Verification items for the finished model (mm, model axes). A direction names the side the tool comes from. Give positions to 0.01 mm unless a question says otherwise; leave off trailing zeros. Order: outer loops, then holes, each group sorted by start corner. A loop starts at its lowest first (then second) coordinate and runs counter-clockwise, first axis right, second up. Notation, with made-up numbers: (39.25, -11.5) -> (62.25, -11.5) arc R36 ccw to (62.25, 23.5) -> close; hole circle Ø10 at (-38, 42.25). An arc over 180 degrees is marked (long way). Write each question's results on one line, items separated by ' | '. Start each with the question number.
1. Material ranges on L1, parallel to X at y = 84, z = 10; L2, parallel to Z at x = 135, y = 82.7; L3, parallel to X at y = 83.7, z = 14, recorded low to high. Write a range as from..to.
2. Cross-section at C-C, the plane x = 135. Enter the section's corners in (y, z).
3. Cross-section at B-B, the plane y = 113.5. Enter the section's corners in (x, z), then the cut area to 3 significant figures.
4. Mould release check, pull along Z, two halves, no side actions. Record for faces 6 (the face through (116.233, 83.268, 4.659)), 7 (the face through (101.039, 127.719, -20.594)), 8 (the face through (139, 106, -3)): +Z half, -Z half, draft (parallel to the pull), parting line (faces both ways), or undercut.
5. Cross-section at D-D, the plane z = 6. Enter the section's corners in (x, y).
6. Depth check by flat-ended pin: pin 1 Ø8 at (x, z) = (135, 6) entering from +Y; pin 2 Ø1.5 at (x, y) = (92.5, 122.5) entering from +Z; pin 3 Ø1.5 at (x, y) = (100.5, 83.5) entering from -Z. Enter the tip coordinate at first touch or a pass-through.
7. Set-up check for faces 1 (the face through (100, 122, -5)), 2 (the face through (125, 123, -21)), 3 (the face through (71.5, 83, 14)), 4 (the face through (63.014, 86.423, -14.499)), 5 (the face through (129, 83, -5)): record each of +Z, -Z, +X, -X, +Y, -Y from which the full face is reachable in a straight line by a thin tool's end or side.
8. Cross-section at A-A, the plane z = -9. Enter the section's corners in (x, y), then the cut area to 3 significant figures.
from build123d import *

# Parameters (mm, degrees)
CYLINDER027_R               = 4
CYLINDER027_DEPTH           = 2.5
CYLINDER027_ROLL_ANGLE      = 90
BOX036_W                    = 14
BOX036_H                    = 10
BOX036_DEPTH                = 11
CYLINDER023_R               = 1.25
CYLINDER023_DEPTH           = 15
CYLINDER023_ROLL_ANGLE      = 90
CYLINDER024_R               = 1.25
CYLINDER024_DEPTH           = 15
CYLINDER024_ROLL_ANGLE      = 90
CYLINDER018_R               = 3.5
CYLINDER018_DEPTH           = 10
CYLINDER019_R               = 3.5
CYLINDER019_DEPTH           = 10
FUSION020_ROLL_ANGLE        = 90
CYLINDER021_R               = 3.5
CYLINDER021_DEPTH           = 10
CYLINDER020_R               = 3.5
CYLINDER020_DEPTH           = 10
FUSION022_ROLL_ANGLE        = 90
BOX018_W                    = 5
BOX018_H                    = 3
BOX018_DEPTH                = 10
BOX035_W                    = 5
BOX035_H                    = 3
BOX035_DEPTH                = 10
BOX025_W                    = 20
BOX025_H                    = 10
BOX025_DEPTH                = 5
BOX024_W                    = 10
BOX024_H                    = 10
BOX024_DEPTH                = 28
FILLET010_R                 = 4.99
BOX022_W                    = 6
BOX022_H                    = 3
BOX022_DEPTH                = 3
CHAMFER002_SIZE             = 2.99
BOX020_W                    = 6
BOX020_H                    = 3
BOX020_DEPTH                = 3
CHAMFER_SIZE                = 2.99
BOX010_W                    = 73
BOX010_H                    = 10
BOX010_DEPTH                = 8
BOX002_W                    = 73
BOX002_H                    = 37
BOX002_DEPTH                = 40
BOX_W                       = 77
BOX_H                       = 48
BOX_DEPTH                   = 40
FILLET_R                    = 8
CYLINDER001_R               = 7
CYLINDER001_DEPTH           = 2
CYLINDER001_PLACEMENT_ANGLE = 29.99999
CYLINDER_R                  = 6
CYLINDER_DEPTH              = 10
CYLINDER_PLACEMENT_ANGLE    = 29.99999
FUSION004_ROLL_ANGLE        = 180
FUSION004_PITCH_ANGLE       = -70
FUSION004_PLACEMENT_ANGLE   = -90


with BuildPart() as cylinder027:
    # Cylinder027 → Cylinder027 (new body)
    with BuildSketch(Plane.XY):
        Circle(CYLINDER027_R)
    extrude(amount=CYLINDER027_DEPTH)


with BuildPart() as cylinder027_1:
    # Cylinder027 roll: moved
    add(cylinder027.part.rotate(Axis((0, 0, 0), (1, 0, 0)), CYLINDER027_ROLL_ANGLE))


with BuildPart() as cylinder027_2:
    # Cylinder027 placement: moved
    add(cylinder027_1.part.moved(Location((63, 84.5, -17))))


with BuildPart() as cube:
    # Box036 → Box036 (new body)
    with BuildSketch(Plane(origin=(129, 78, -10), x_dir=(1, 0, 0), z_dir=(0, 0, 1))):
        with Locations((7, 5)):
            Rectangle(BOX036_W, BOX036_H)
    extrude(amount=BOX036_DEPTH)


with BuildPart() as cylinder023:
    # Cylinder023 → Cylinder023 (new body)
    with BuildSketch(Plane.XY):
        Circle(CYLINDER023_R)
    extrude(amount=CYLINDER023_DEPTH)


with BuildPart() as cylinder023_1:
    # Cylinder023 roll: moved
    add(cylinder023.part.rotate(Axis((0, 0, 0), (1, 0, 0)), CYLINDER023_ROLL_ANGLE))


with BuildPart() as cylinder023_2:
    # Cylinder023 placement: moved
    add(cylinder023_1.part.moved(Location((74, 97, 10))))


with BuildPart() as fusion031:
    # Cylinder024 → Cylinder024 (new body)
    with BuildSketch(Plane.XY):
        Circle(CYLINDER024_R)
    extrude(amount=CYLINDER024_DEPTH)


with BuildPart() as fusion031_1:
    # Cylinder024 roll: moved
    add(fusion031.part.rotate(Axis((0, 0, 0), (1, 0, 0)), CYLINDER024_ROLL_ANGLE))


with BuildPart() as fusion031_2:
    # Cylinder024 placement: moved
    add(fusion031_1.part.moved(Location((106, 97, 10))))

    # Fusion031: union Cylinder023
    add(cylinder023_2.part)


with BuildPart() as fusion031_3:
    # Fusion031 placement: moved
    add(fusion031_2.part.moved(Location((0, -8, 0))))


with BuildPart() as cylinder018:
    # Cylinder018 → Cylinder018 (new body)
    with BuildSketch(Plane(origin=(-8, 25.5, 0), x_dir=(1, 0, 0), z_dir=(0, 0, 1))):
        Circle(CYLINDER018_R)
    extrude(amount=CYLINDER018_DEPTH)


with BuildPart() as fusion020:
    # Cylinder019 → Cylinder019 (new body)
    with BuildSketch(Plane(origin=(-8, 33.5, 0), x_dir=(1, 0, 0), z_dir=(0, 0, 1))):
        Circle(CYLINDER019_R)
    extrude(amount=CYLINDER019_DEPTH)

    # Fusion020: union Cylinder018
    add(cylinder018.part)


with BuildPart() as fusion020_1:
    # Fusion020 roll: moved
    add(fusion020.part.rotate(Axis((0, 0, 0), (1, 0, 0)), FUSION020_ROLL_ANGLE))


with BuildPart() as fusion020_2:
    # Fusion020 placement: moved
    add(fusion020_1.part.moved(Location((312, 84.5, -19.5))))


with BuildPart() as cylinder021:
    # Cylinder021 → Cylinder021 (new body)
    with BuildSketch(Plane(origin=(-8, 25.5, 0), x_dir=(1, 0, 0), z_dir=(0, 0, 1))):
        Circle(CYLINDER021_R)
    extrude(amount=CYLINDER021_DEPTH)


with BuildPart() as fusion023:
    # Cylinder020 → Cylinder020 (new body)
    with BuildSketch(Plane(origin=(-8, 33.5, 0), x_dir=(1, 0, 0), z_dir=(0, 0, 1))):
        Circle(CYLINDER020_R)
    extrude(amount=CYLINDER020_DEPTH)

    # Fusion022: union Cylinder021
    add(cylinder021.part)


with BuildPart() as fusion023_1:
    # Fusion022 roll: moved
    add(fusion023.part.rotate(Axis((0, 0, 0), (1, 0, 0)), FUSION022_ROLL_ANGLE))


with BuildPart() as fusion023_2:
    # Fusion022 placement: moved
    add(fusion023_1.part.moved(Location((334, 84.5, -19.5))))

    # Fusion023: union Fusion020
    add(fusion020_2.part)


with BuildPart() as fusion023_3:
    # Fusion023 placement: moved
    add(fusion023_2.part.moved(Location((-191, 0, 0))))


with BuildPart() as box018:
    # Box018 → Box018 (new body)
    with BuildSketch(Plane(origin=(71.5, 82, 5), x_dir=(1, 0, 0), z_dir=(0, 0, 1))):
        with Locations((2.5, 1.5)):
            Rectangle(BOX018_W, BOX018_H)
    extrude(amount=BOX018_DEPTH)


with BuildPart() as box035:
    # Box035 → Box035 (new body)
    with BuildSketch(Plane(origin=(103.5, 82, 5), x_dir=(1, 0, 0), z_dir=(0, 0, 1))):
        with Locations((2.5, 1.5)):
            Rectangle(BOX035_W, BOX035_H)
    extrude(amount=BOX035_DEPTH)


with BuildPart() as box025:
    # Box025 → Box025 (new body)
    with BuildSketch(Plane(origin=(90, 112, 9), x_dir=(1, 0, 0), z_dir=(0, 0, 1))):
        with Locations((10, 5)):
            Rectangle(BOX025_W, BOX025_H)
    extrude(amount=BOX025_DEPTH)


with BuildPart() as fillet010:
    # Box024 → Box024 (new body)
    with BuildSketch(Plane(origin=(54, 85, -16), x_dir=(1, 0, 0), z_dir=(0, 0, 1))):
        with Locations((5, 5)):
            Rectangle(BOX024_W, BOX024_H)
    extrude(amount=BOX024_DEPTH)

    # Fillet010
    fillet010_edges = [fillet010.edges().sort_by_distance(p)[0] for p in [
        (59, 85, -16),
        (59, 85, 12),
        (59, 95, -16),
        (59, 95, 12),
    ]]
    fillet(fillet010_edges, radius=FILLET010_R)


with BuildPart() as chamfer002:
    # Box022 → Box022 (new body)
    with BuildSketch(Plane(origin=(70, 113, -23), x_dir=(1, 0, 0), z_dir=(0, 0, 1))):
        with Locations((3, 1.5)):
            Rectangle(BOX022_W, BOX022_H)
    extrude(amount=BOX022_DEPTH)

    # Chamfer002
    chamfer002_edges = [chamfer002.edges().sort_by_distance(p)[0] for p in [
        (73, 116, -23),
    ]]
    chamfer(chamfer002_edges, length=CHAMFER002_SIZE)


with BuildPart() as chamfer002_1:
    # Chamfer002 placement: moved
    add(chamfer002.part.moved(Location((55, 9, 0.5))))


with BuildPart() as fusion028:
    # Box020 → Box020 (new body)
    with BuildSketch(Plane(origin=(70, 113, -23), x_dir=(1, 0, 0), z_dir=(0, 0, 1))):
        with Locations((3, 1.5)):
            Rectangle(BOX020_W, BOX020_H)
    extrude(amount=BOX020_DEPTH)

    # Chamfer
    chamfer_edges = [fusion028.edges().sort_by_distance(p)[0] for p in [
        (73, 116, -23),
    ]]
    chamfer(chamfer_edges, length=CHAMFER_SIZE)


with BuildPart() as fusion028_1:
    # Chamfer placement: moved
    add(fusion028.part.moved(Location((1, 9, 0.5))))

    # Fusion028: union Chamfer002
    add(chamfer002_1.part)


with BuildPart() as box010:
    # Box010 → Box010 (new body)
    with BuildSketch(Plane(origin=(64, 82, -23), x_dir=(1, 0, 0), z_dir=(0, 0, 1))):
        with Locations((36.5, 5)):
            Rectangle(BOX010_W, BOX010_H)
    extrude(amount=BOX010_DEPTH)


with BuildPart() as box002:
    # Box002 → Box002 (new body)
    with BuildSketch(Plane(origin=(64, 85, -26), x_dir=(1, 0, 0), z_dir=(0, 0, 1))):
        with Locations((36.5, 18.5)):
            Rectangle(BOX002_W, BOX002_H)
    extrude(amount=BOX002_DEPTH)


with BuildPart() as cut019:
    # Box → Box (new body)
    with BuildSketch(Plane(origin=(62, 82, -27), x_dir=(1, 0, 0), z_dir=(0, 0, 1))):
        with Locations((38.5, 24)):
            Rectangle(BOX_W, BOX_H)
    extrude(amount=BOX_DEPTH)

    # Fillet
    fillet_edges = [cut019.edges().sort_by_distance(p)[0] for p in [
        (100.5, 82, -27),
        (100.5, 82, 13),
        (100.5, 130, -27),
        (100.5, 130, 13),
    ]]
    fillet(fillet_edges, radius=FILLET_R)


with BuildPart() as cut019_1:
    # Fillet placement: moved
    add(cut019.part.moved(Location((0, 0, 4))))

    # Cut001: cut Box002
    add(box002.part, mode=Mode.SUBTRACT)

    # Cut004: cut Box010
    add(box010.part, mode=Mode.SUBTRACT)

    # Cut018: cut Fusion028
    add(fusion028_1.part, mode=Mode.SUBTRACT)

    # Cut019: cut Fillet010
    add(fillet010.part, mode=Mode.SUBTRACT)


with BuildPart() as cylinder001:
    # Cylinder001 → Cylinder001 (new body)
    with BuildSketch(Plane.XY):
        Circle(CYLINDER001_R)
    extrude(amount=CYLINDER001_DEPTH)


with BuildPart() as cylinder001_1:
    # Cylinder001 placement: moved
    add(cylinder001.part.moved(Location((51, 75, -3))).rotate(Axis((51, 75, -3), (0, -1, 0)), CYLINDER001_PLACEMENT_ANGLE))


with BuildPart() as cut025:
    # Cylinder → Cylinder (new body)
    with BuildSketch(Plane.XY):
        Circle(CYLINDER_R)
    extrude(amount=CYLINDER_DEPTH)


with BuildPart() as cut025_1:
    # Cylinder placement: moved
    add(cut025.part.moved(Location((51, 75, -3))).rotate(Axis((51, 75, -3), (0, -1, 0)), CYLINDER_PLACEMENT_ANGLE))

    # Fusion004: union Cylinder001
    add(cylinder001_1.part)


with BuildPart() as cut025_2:
    # Fusion004 roll: moved
    add(cut025_1.part.rotate(Axis((0, 0, 0), (1, 0, 0)), FUSION004_ROLL_ANGLE))


with BuildPart() as cut025_3:
    # Fusion004 pitch: moved
    add(cut025_2.part.rotate(Axis((0, 0, 0), (0, 1, 0)), FUSION004_PITCH_ANGLE))


with BuildPart() as cut025_4:
    # Fusion004 placement: moved
    add(cut025_3.part.moved(Location((175.5, 143.464742, -29.748779))).rotate(Axis((175.5, 143.464742, -29.748779), (0, 0, 1)), FUSION004_PLACEMENT_ANGLE))

    # Fusion029: union Cut019
    add(cut019_1.part)

    # Cut020: cut Box025
    add(box025.part, mode=Mode.SUBTRACT)

    # Fusion030: union Box018, Box035
    add(box018.part)
    add(box035.part)

    # Cut021: cut Fusion023
    add(fusion023_3.part, mode=Mode.SUBTRACT)

    # Cut022: cut Fusion031
    add(fusion031_3.part, mode=Mode.SUBTRACT)

    # Cut023: cut Cube
    add(cube.part, mode=Mode.SUBTRACT)

    # Cut025: cut Cylinder027
    add(cylinder027_2.part, mode=Mode.SUBTRACT)


solid = cut025_4.part
Results below:
1) L1: x = 62..72.75, 75.25..104.75, 107.25..139 | L2: z = -15..-10, 1..2.5, 9.5..10.5 | L3: x = 71.5..76.5, 103.5..108.5
2) outline: (82, -15) -> (85, -15) -> (85, -10) -> (82, -10) -> close; (82, 1) -> (85, 1) -> (85, 14) -> (122, 14) -> (122, -23) arc R8 ccw to (130, -15) -> (130, 9) arc R8 ccw to (122, 17) -> (90, 17) arc R8 ccw to (84.5, 14.81) -> (84.5, 10.5) -> (82.14, 10.5) arc R8 ccw to (82.02, 9.5) -> (84.5, 9.5) -> (84.5, 2.5) -> (82, 2.5) -> close
3) outline: (62, -23) -> (64, -23) -> (64, 14) -> (137, 14) -> (137, -23) -> (139, -23) -> (139, 17) -> (62, 17) -> close | area: 379 mm²
4) face 6: undercut | face 7: -Z half | face 8: draft
5) outline: (62, 82) -> (109.5, 82) -> (109.5, 84.5) -> (116.5, 84.5) -> (116.5, 82) -> (131.5, 82) -> (131.5, 84.5) -> (138.5, 84.5) -> (138.5, 82) -> (139, 82) -> (139, 130) -> (62, 130) -> (62, 95) -> (64, 95) -> (64, 122) -> (137, 122) -> (137, 85) -> (62, 85) -> close
6) pin 1: stops at y = 130 | pin 2: stops at z = 17 | pin 3: stops at z = -15
7) face 1: -Z | face 2: -Y | face 3: +Z, -X, -Y | face 4: -X | face 5: +X, -Y
8) outline: (62, 82) -> (129, 82) -> (129, 85) -> (62, 85) -> close; (62, 95) -> (64, 95) -> (64, 122) -> (137, 122) -> (137, 88) -> (139, 88) -> (139, 130) -> (62, 130) -> close | area: 939 mm²
